Here's how the part is built. I have some questions about the finished solid (model axes, mm). Face numbers are marked on the shaded views. A direction names the side the tool comes from. Coordinates: 2 decimals unless noted, no trailing zeros. Write each loop counter-clockwise with the first axis right and the second up, starting at its lowest first coordinate (ties: lowest second). Pieces come first, ordered by that corner, then holes.
Item 1: We'd pull the mould along X, two halves only. Please class the marked faces 4, 5 and 6: +X half, -X half, draft (parallel to the pull), parting line (faces both ways), or undercut.
Item 2: For the marked faces 1, 2 and 3, which set-ups out of +Z, -Z, +X, -X, +Y, -Y let a thin tool reach every point of the face, with its end or its side?
Item 3: If I drill on line 1 (X direction, y = 5, z = -16); line 2 (Y direction, x = 4, z = -15); line 3 (Y direction, x = -2.7, z = -23.75), over which ranges is the centre line in solid material (lowest first)?
Item 4: If we section it at B-B (z = -9): Please give me the cut outline in (x, y), then the cut area to 3 significant figures.
Item 5: I'm going to push flat-ended pins straight in: pin 1 Ø4.5 at (y, z) = (13.94, -23.75) entering from +X; pin 2 Ø3 at (y, z) = (15.5, 3) entering from +X; pin 3 Ø8.5 at (y, z) = (6.5, -6.5) entering from -X; pin 4 Ø3 at (x, y) = (2, 13) entering from +Z. Where does each tip first touch, or does it pass through?
Item 6: If we section it at C-C (x = 1.5): Please give me the cut outline in (y, z).
Item 7: If we section it at A-A (x = -0.5): Please give me the cut outline in (y, z), then the cut area to 3 significant figures.
Item 8: If we section it at D-D (z = -17.5): Please give me the cut outline in (x, y).
from build123d import *

# Parameters (mm, degrees)
SKETCH2_W               = 17.75
SKETCH2_H               = 20.7
SKETCH2_R               = 1.22
BOSS_EXTRUDE1_DEPTH     = 1.5
CUT_EXTRUDE2_START      = -10.5
CUT_EXTRUDE2_OUTLINE_W  = 20.7
CUT_EXTRUDE2_OUTLINE_H  = 1.5
CUT_EXTRUDE2_DEPTH      = 10.5
SKETCH5_W               = 20.7
SKETCH5_H               = 8.940198937
BOSS_EXTRUDE3_DEPTH     = 1.5
BOSS_EXTRUDE5_OUTLINE_W = 1.5
BOSS_EXTRUDE5_OUTLINE_H = 20.7
BOSS_EXTRUDE5_DEPTH     = 4.5
SKETCH26_W              = 33.7
SKETCH26_H              = 6.9
SKETCH26_R              = 1.35
BOSS_EXTRUDE9_DEPTH     = 3
CUT_EXTRUDE3_DEPTH      = 0.55
CUT_EXTRUDE3_DEPTH_BACK = 1.5


# Read off the part's stored shape, not the designer's step: Cut-Extrude2, Boss-Extrude5
with BuildPart() as part:
    # Sketch2 → Boss-Extrude1 (new body)
    with BuildSketch(Plane(origin=(0, 0, 0), x_dir=(1, 0, 0), z_dir=(0, 1, 0))):
        with Locations((8.875, 10.35)):
            Rectangle(SKETCH2_W, SKETCH2_H)
        with Locations(Location((1.996494824, 2.32830664, 0), (0, 0, 270))):
            Circle(SKETCH2_R, mode=Mode.SUBTRACT)
        with Locations(Location((1.982091411, 18.38849058, 0), (0, 0, 270))):
            Circle(SKETCH2_R, mode=Mode.SUBTRACT)
    extrude(amount=BOSS_EXTRUDE1_DEPTH)

    # Cut-Extrude2 outline → Cut-Extrude2 (cut)
    with BuildSketch(Plane(origin=(17.75, 0, 0), x_dir=(0, 0, -1), z_dir=(1, 0, 0)).offset(CUT_EXTRUDE2_START)):
        with Locations((10.35, 0.75)):
            Rectangle(CUT_EXTRUDE2_OUTLINE_W, CUT_EXTRUDE2_OUTLINE_H)
    extrude(amount=CUT_EXTRUDE2_DEPTH, mode=Mode.SUBTRACT)

    # Sketch5 → Boss-Extrude3 (add)
    with BuildSketch(Plane.ZY):
        with Locations((-10.35, 4.470099468)):
            Rectangle(SKETCH5_W, SKETCH5_H)
    extrude(amount=BOSS_EXTRUDE3_DEPTH)

    # Boss-Extrude5 outline → Boss-Extrude5 (add)
    with BuildSketch(Plane(origin=(0, 8.940198937, 0), x_dir=(1, 0, 0), z_dir=(0, 1, 0))):
        with Locations((-0.75, 10.35)):
            Rectangle(BOSS_EXTRUDE5_OUTLINE_W, BOSS_EXTRUDE5_OUTLINE_H)
    extrude(amount=BOSS_EXTRUDE5_DEPTH)

    # Sketch26 → Boss-Extrude9 (add)
    with BuildSketch(Plane(origin=(0, 0, 0), x_dir=(0, 0, -1), z_dir=(1, 0, 0))):
        with Locations((10.35, 13.940198937)):
            Rectangle(SKETCH26_W, SKETCH26_H)
        with Locations((23.75, 13.940198937)):
            Circle(SKETCH26_R, mode=Mode.SUBTRACT)
        with Locations((-3.05, 13.940198937)):
            Circle(SKETCH26_R, mode=Mode.SUBTRACT)
    extrude(amount=-BOSS_EXTRUDE9_DEPTH)

    # Sketch29 → Cut-Extrude3 (cut, two sides: drawn at the far end of the back side and taken through both)
    with BuildSketch(Plane.ZY.offset(1.5).offset(-CUT_EXTRUDE3_DEPTH_BACK)):
        Polygon((-26.5, 12.352485697), (-23.75, 10.764772456), (-21, 12.352485697), (-21, 15.527912177), (-23.75, 17.115625417), (-26.5, 15.527912177), align=None)
        Polygon((0.3, 12.352485697), (3.05, 10.764772456), (5.8, 12.352485697), (5.8, 15.527912177), (3.05, 17.115625417), (0.3, 15.527912177), align=None)
    extrude(amount=CUT_EXTRUDE3_DEPTH + CUT_EXTRUDE3_DEPTH_BACK, mode=Mode.SUBTRACT)


solid = part.part
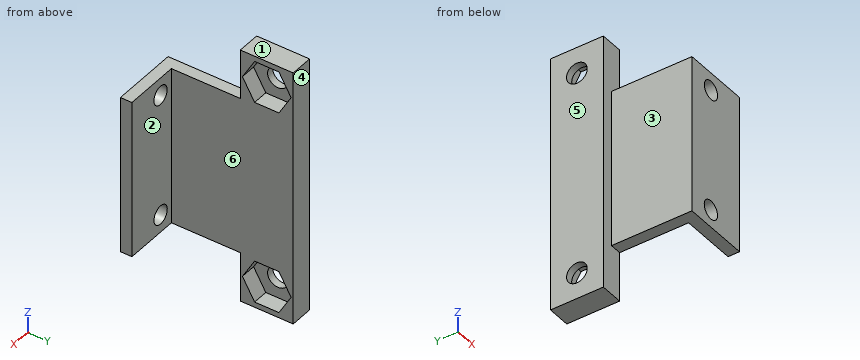
Answer list:
1. face 4: draft
1. face 5: -X half
1. face 6: +X half
2. face 1: +Z, +X, -X, +Y, -Y
2. face 2: +Z, -Z, +X, +Y
2. face 3: +Z, -Z, -X, -Y
3. line 1: x = -1.5 to 0
3. line 2: y = 0 to 1.5
3. line 3: y = 10.49 to 12.59, 15.29 to 17.39
4. outline: (-3, 10.49) - (-1.5, 10.49) - (-1.5, 0) - (7.25, 0) - (7.25, 1.5) - (0, 1.5) - (0, 17.39) - (-3, 17.39) - close
4. area: 47.3 mm2
5. pin 1: stops at x = -2.05
5. pin 2: stops at x = 0
5. pin 3: stops at x = -3
5. pin 4: passes through
6. outline: (0, -20.7) - (1.5, -20.7) - (1.5, -19.51) - (0, -19.51) - close; (0, -17.27) - (1.5, -17.27) - (1.5, -3.44) - (0, -3.44) - close; (0, -1.21) - (1.5, -1.21) - (1.5, 0) - (0, 0) - close
7. outline: (0, -20.7) - (10.49, -20.7) - (10.49, -27.2) - (17.39, -27.2) - (17.39, 6.5) - (10.49, 6.5) - (10.49, 0) - (0, 0) - close; hole (10.76, -23.75) - (12.35, -26.5) - (15.53, -26.5) - (17.12, -23.75) - (15.53, -21) - (12.35, -21) - close; hole (10.76, 3.05) - (12.35, 0.3) - (15.53, 0.3) - (17.12, 3.05) - (15.53, 5.8) - (12.35, 5.8) - close
7. area: 397 mm2
8. outline: (-3, 10.49) - (-1.5, 10.49) - (-1.5, 0) - (1.15, 0) - (1.15, 1.5) - (0, 1.5) - (0, 17.39) - (-3, 17.39) - close; (2.82, 0) - (7.25, 0) - (7.25, 1.5) - (2.82, 1.5) - close
